from build123d import *

# Parameters (mm, degrees)
BOSS_EXTRUDE1_DEPTH     = 17
CUT_EXTRUDE3_DEPTH      = 27
CUT_EXTRUDE3_DEPTH_BACK = 17
SKETCH5_W               = 9.47
SKETCH5_H               = 10.75
CUT_EXTRUDE4_REACH      = 35.912
SKETCH7_W               = 10
SKETCH7_H               = 10.75
SKETCH8_R               = 4
CUT_EXTRUDE5_DEPTH      = 37


with BuildPart() as part:
    # Sketch1 → Boss-Extrude1 (new body)
    with BuildSketch(Plane.XY):
        Polygon((-13.217142857, 28.337142857), (-8.177142857, 28.337142857), (-8.177142857, 17.237142857), (11.505594759, 17.237142857), (11.505594759, 28.337142857), (16.545594759, 28.337142857), (16.545594759, 10.516618894), (14.225387594, 5.673733524), (-4.003880739, -6.9964589), (-9, -2.622857143), (-13.217142857, 13.337142857), align=None)
    extrude(amount=BOSS_EXTRUDE1_DEPTH)

    # Sketch4 → Cut-Extrude3 (cut, two sides: drawn at the far end of the back side and taken through both)
    with BuildSketch(Plane(origin=(-8.177142857, 0, 0), x_dir=(0, 0, -1), z_dir=(1, 0, 0)).offset(-CUT_EXTRUDE3_DEPTH_BACK)):
        with BuildLine():
            Line((-17, 28.337142857), (-17, 17.4025989))
            ThreePointArc((-17, 17.4025989), (-14.6995428, 24.220877118), (-8.797223125, 28.337142857))
            Line((-8.797223125, 28.337142857), (-17, 28.337142857))
        make_face()
        Polygon((-3.797223125, 27.774535639), (0, 23.997142857), (0, 28.337142857), (-8.797223125, 28.337142857), align=None)
    extrude(amount=CUT_EXTRUDE3_DEPTH + CUT_EXTRUDE3_DEPTH_BACK, mode=Mode.SUBTRACT)

    # Cut-Sweep1: sweep along a path in Sketch6
    with BuildLine(Plane.XY.offset(10)) as cut_sweep1_path:
        Line((0.85151547, -3.621731888), (-5.920332926, 2.306342783))
    # Sketch5 → Cut-Sweep1 (sweep, cut)
    with BuildSketch(Plane(origin=(1.974682223, -2.841078565, 0), x_dir=(0.8211382131865097, 0.5707293884538155, 0), z_dir=(0.5707293884538155, -0.8211382131865098, 0))):
        with Locations((1.454175815, 7.885)):
            Rectangle(SKETCH5_W, SKETCH5_H)
    sweep(path=cut_sweep1_path.line, mode=Mode.SUBTRACT)

    # Cut-Extrude4: up to this face of the body (flat: up to its plane)
    cut_extrude4_end = Plane(part.part.faces().sort_by_distance((-4.105252084, -1.749504011, 7.885))[0])
    # Sketch7 → Cut-Extrude4 (cut, up to the picked face)
    with BuildSketch(Plane(origin=(0, 17.237142857, 0), x_dir=(1, 0, 0), z_dir=(0, 1, 0)), mode=Mode.PRIVATE) as cut_extrude4_sk1:
        with Locations((0.242857143, -7.885)):
            Rectangle(SKETCH7_W, SKETCH7_H)
    cut_extrude4_tool1 = split(extrude(cut_extrude4_sk1.sketch, amount=-CUT_EXTRUDE4_REACH, mode=Mode.PRIVATE), bisect_by=cut_extrude4_end, keep=Keep.BOTH, mode=Mode.PRIVATE)
    add(cut_extrude4_tool1.solids().sort_by(Axis((0.242857, 17.237143, 7.885), (0, -1, 0)))[0], mode=Mode.SUBTRACT)

    # Sketch8 → Cut-Extrude5 (cut)
    with BuildSketch(Plane.ZY.offset(13.217142857)):
        with Locations(Location((9, 21.937142857, 0), (0, 0, 90))):
            Circle(SKETCH8_R)
    extrude(amount=-CUT_EXTRUDE5_DEPTH, mode=Mode.SUBTRACT)


solid = part.part
Verification items for the finished model (mm, model axes). A direction names the side the tool comes from. Coordinates: 2 decimals unless noted, no trailing zeros. Order: outer loops, then holes, each group sorted by start corner. A loop starts at its lowest first (then second) coordinate and runs counter-clockwise, first axis right, second up.
Item 1: Access from +Z, -Z, +X, -X, +Y, -Y to the whole of each face (thin tool, end or side, straight path). Record for faces 1 (the face through (5.243, 10, 8)), 2 (the face through (13.99, 24.14, 14.76)), 3 (the face through (11.506, 22.7, 4.6)).
Filled in:
face 1: +Y, -Y
face 2: +Z, +X, -X, +Y
face 3: +Z, -Z, +Y
Item 2: Section check C-C, the plane z = 11.25. Enter the section's corners in (x, y), then the cut area to 3 significant figures.
Filled in:
outline: (-13.22, 13.34) - (-9, -2.62) - (-4, -7) - (-0.72, -4.71) - (-7.49, 1.21) - (-4.76, 3.11) - (-4.76, 17.24) - (-8.18, 17.24) - (-8.18, 18.63) - (-13.22, 18.63) - close; (-13.22, 25.24) - (-8.18, 25.24) - (-8.18, 27.28) - (-13.22, 27.28) - close; (5.24, 2.28) - (7.06, 0.69) - (14.23, 5.67) - (16.55, 10.52) - (16.55, 18.63) - (11.51, 18.63) - (11.51, 17.24) - (5.24, 17.24) - close; (11.51, 25.24) - (16.55, 25.24) - (16.55, 27.28) - (11.51, 27.28) - close
area: 334 mm2
Item 3: Release check for a two-part mould opening along Y. For faces 4 (the face through (-6.105, 2.178, 7.81)), 5 (the face through (6.137, 1.496, 7.81)), 6 (the face through (-13.217, 17, 8)) record: +Y half, -Y half, draft (parallel to the pull), parting line (faces both ways), or undercut.
Filled in:
face 4: undercut
face 5: -Y half
face 6: draft
Item 4: Depth check by flat-ended pin: pin 1 (10 mm diameter, centred on x = -10, z = 14, fed in from +Y); pin 2 (4 mm diameter, centred on x = -8.5, z = 10.5, fed in from -Y); pin 3 (5.5 mm diameter, centred on y = 7.5, z = 8, fed in from -X). Enter the tip coordinate at first touch or a pass-through.
Filled in:
pin 1: stops at y = 28.27
pin 2: stops at y = -4.81
pin 3: stops at x = -12.4
Item 5: Material ranges on L1, parallel to X at y = 19, z = 5.5; L2, parallel to Z at x = 13, y = 18.5; L3, parallel to X at y = 1, z = 5.75, recorded low to high.
Filled in:
L1: x = -13.22 to -8.18, 11.51 to 16.55
L2: z = 0 to 6.95, 11.05 to 16.94
L3: x = -9.96 to -7.25, 6.7 to 7.5
Item 6: Section check B-B, the plane x = 1. Enter the section's corners in (y, z), then the cut area to 3 significant figures.
Filled in:
outline: (-3.52, 0) - (17.24, 0) - (17.24, 2.51) - (-3.52, 2.51) - close; (-3.52, 13.26) - (17.24, 13.26) - (17.24, 17) - (-3.52, 17) - close
area: 130 mm2
Item 7: Section check A-A, the plane y = 15. Enter the section's corners in (x, z).
Filled in:
outline: (-13.22, 0) - (16.55, 0) - (16.55, 17) - (-13.22, 17) - close; hole (-4.76, 2.51) - (5.24, 2.51) - (5.24, 13.26) - (-4.76, 13.26) - close
Item 8: Section check D-D, the plane y = 20.5. Enter the section's corners in (x, z), then the cut area to 3 significant figures.
Filled in:
outline: (-13.22, 0) - (-8.18, 0) - (-8.18, 5.27) - (-13.22, 5.27) - close; (-13.22, 12.73) - (-8.18, 12.73) - (-8.18, 16.55) - (-13.22, 16.55) - close; (11.51, 0) - (16.55, 0) - (16.55, 5.27) - (11.51, 5.27) - close; (11.51, 12.73) - (16.55, 12.73) - (16.55, 16.55) - (11.51, 16.55) - close
area: 91.6 mm2
